Study the drawing (mm; zero at the part's minimum x, y, z) and answer. A direction names the side the tool comes from. Round coordinates to 2 decimals unless told otherwise and drop trailing zeros. Write each loop counter-clockwise with the first axis right and the second up, starting at its lowest first coordinate (ties: lowest second). Pieces come first, ordered by that corner, then holes.
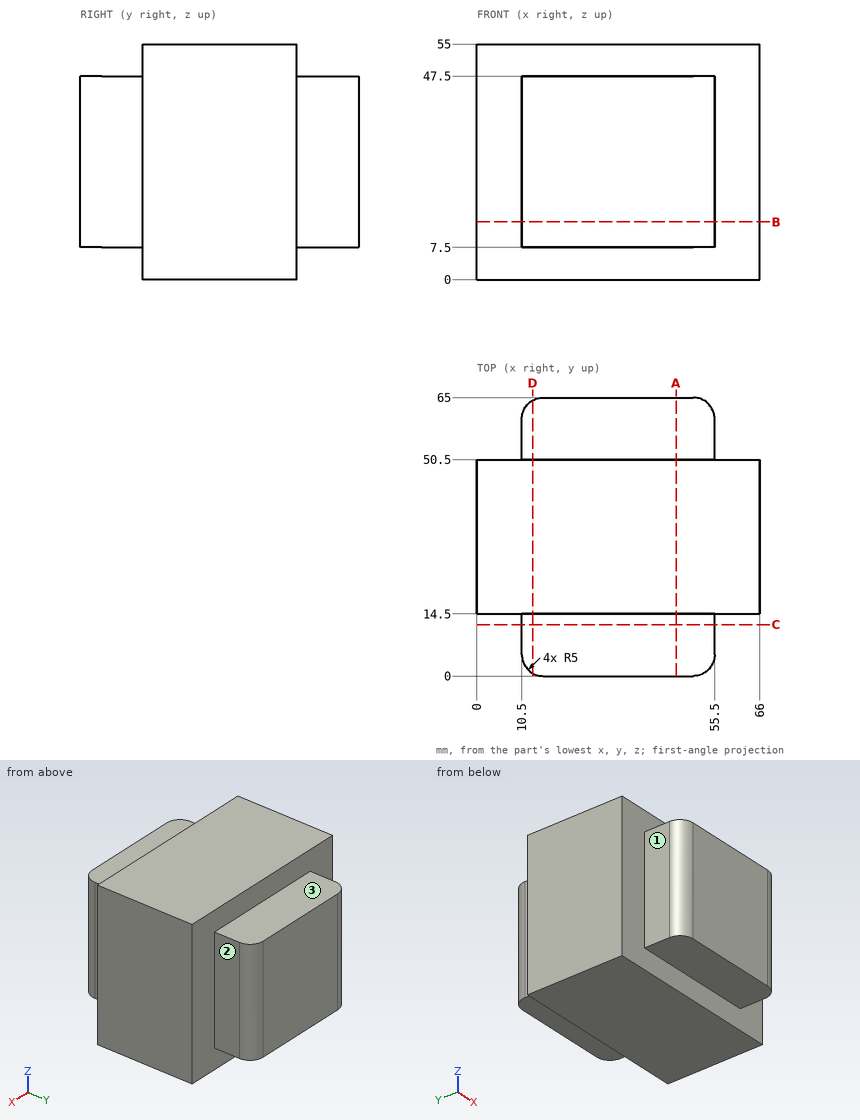
1. Section B-B on z = 13.5 is taken. Determine the outline of the cut face in (x, y).
Geometry says:
outline: (0, 14.5) - (10.5, 14.5) - (10.5, 5) arc R5 ccw to (15.5, 0) - (50.5, 0) arc R5 ccw to (55.5, 5) - (55.5, 14.5) - (66, 14.5) - (66, 50.5) - (55.5, 50.5) - (55.5, 60) arc R5 ccw to (50.5, 65) - (15.5, 65) arc R5 ccw to (10.5, 60) - (10.5, 50.5) - (0, 50.5) - close
2. Section D-D on x = 13 is taken. Determine the outline of the cut face in (y, z), plus the area to 3 significant figures.
Geometry says:
outline: (0.67, 7.5) - (14.5, 7.5) - (14.5, 0) - (50.5, 0) - (50.5, 7.5) - (64.33, 7.5) - (64.33, 47.5) - (50.5, 47.5) - (50.5, 55) - (14.5, 55) - (14.5, 47.5) - (0.67, 47.5) - close
area: 3,090 mm2
3. Given pin 1 (1.5 mm diameter, centred on x = 58.5, z = 47, fed in from -Y); pin 2 (7 mm diameter, centred on x = 37.5, y = 6, fed in from -Z); pin 3 (4.5 mm diameter, centred on x = 34.5, y = 9, fed in from +Z), each flat-ended and moving along its own axis, determine where each tip first touches the part or whether it passes through.
Geometry says:
pin 1: stops at y = 14.5
pin 2: stops at z = 7.5
pin 3: stops at z = 47.5
4. Section C-C on y = 12 is taken. Determine the outline of the cut face in (x, z).
Geometry says:
outline: (10.5, 7.5) - (55.5, 7.5) - (55.5, 47.5) - (10.5, 47.5) - close
5. Section A-A on x = 46.5 is taken. Determine the outline of the cut face in (y, z).
Geometry says:
outline: (0, 7.5) - (14.5, 7.5) - (14.5, 0) - (50.5, 0) - (50.5, 7.5) - (65, 7.5) - (65, 47.5) - (50.5, 47.5) - (50.5, 55) - (14.5, 55) - (14.5, 47.5) - (0, 47.5) - close
6. Straight lines are drawn through the part: line 1 along Y through (x, z) = (63.5, 10); line 2 along X through (y, z) = (6.5, 38); line 3 along Z through (x, y) = (43, 11.5). For each, find the intervals that lie inside material, in ascending order.
Geometry says:
line 1: y = 14.5 to 50.5
line 2: x = 10.5 to 55.5
line 3: z = 7.5 to 47.5
7. A tool of negligible diameter and unlimited length cuts with its end or side. For the marked faces 1, 2 and 3, from which of +Z, -Z, +X, -X, +Y, -Y can it reach the whole face along a straight path? Write none if from no direction.
Geometry says:
face 1: +Z, -Z, -X, -Y
face 2: +Z, -Z, +X, +Y
face 3: +Z, +X, -X, +Y
